from build123d import *

# Parameters (mm, degrees)
F0_W          = 135.364354
F0_H          = 59.463624
F1_DEPTH      = 25.4
F2_R          = 21.942161
F3_DEPTH      = 25.4
F5_DEPTH      = 25.4
F5_DEPTH_BACK = 25.4


with BuildPart() as f1:
    # F0 (on Front) → F1 (new body)
    with BuildSketch(Plane.XZ):
        Rectangle(F0_W, F0_H)
    extrude(amount=F1_DEPTH)

    # F2 (on face) → F3 (join)
    with BuildSketch(Plane.XZ.offset(25.4)):
        Circle(F2_R)
    extrude(amount=F3_DEPTH)

    # F4 (on Top) → F5 (cut, two sides)
    with BuildSketch(Plane.XY) as f5_sk:
        Polygon((34.163382, -53.259425), (-24.172205, -40.689882), (-24.172205, -53.259425), align=None)
    extrude(amount=F5_DEPTH, mode=Mode.SUBTRACT)
    extrude(f5_sk.sketch, amount=-F5_DEPTH_BACK, mode=Mode.SUBTRACT)


solid = f1.part
Part model, mm, in its own coordinate system. A direction names the side the tool comes from. Give positions to 0.01 mm unless a question says otherwise; leave off trailing zeros. Write each loop counter-clockwise with the first axis right and the second up, starting at its lowest first coordinate (ties: lowest second). Pieces come first, ordered by that corner, then holes.
1) Cut at C-C on x = 0. Write the cut outline in (y, z).
Resolved:
outline: (-45.9, -21.94) - (-25.4, -21.94) - (-25.4, -29.73) - (0, -29.73) - (0, 29.73) - (-25.4, 29.73) - (-25.4, 21.94) - (-45.9, 21.94) - close
2) Probe L1, parallel to Y at x = 29, z = 4; L2, parallel to X at y = -29, z = 0; L3, parallel to X at y = -33.5, z = 7. List the from-to ranges inside material, lowest first.
Resolved:
L1: y = -25.4 to 0
L2: x = -21.94 to 21.94
L3: x = -20.8 to 20.8
3) Cut at A-A on z = 0. Write the cut outline in (x, y).
Resolved:
outline: (-67.68, -25.4) - (-21.94, -25.4) - (-21.94, -41.17) - (21.94, -50.63) - (21.94, -25.4) - (67.68, -25.4) - (67.68, 0) - (-67.68, 0) - close
4) Pin check, flat tips, straight feed: pin 1 (10 mm diameter, centred on x = 48.5, z = -6.5, fed in from -Y); pin 2 (12 mm diameter, centred on x = -5, z = 12, fed in from -Y); pin 3 (6 mm diameter, centred on x = 21, y = -42, fed in from +Z). Stop position of each tip, or through.
Resolved:
pin 1: stops at y = -25.4
pin 2: stops at y = -46.11
pin 3: stops at z = 12.55
5) Cut at D-D on x = -57.5. Write the cut outline in (y, z), then the cut area to 3 significant figures.
Resolved:
outline: (-25.4, -29.73) - (0, -29.73) - (0, 29.73) - (-25.4, 29.73) - close
area: 1,510 mm2
6) Which spindle directions (+Z, -Z, +X, -X, +Y, -Y) get a long thin tool onto all of the face, cutting with end or side? Do faces 1 (the face through (0.307, -45.964, 0.307)), 2 (the face through (20.93, -35.03, 6.59)). Say none if no direction does.
Resolved:
face 1: +Z, -Z, -X, -Y
face 2: -Y
7) Cut at B-B on y = -36. Write the cut outline in (x, z).
Resolved:
outline: circle Ø43.88 at (0, 0)
